Autodesk Inventor part; units mm, degrees
ref_plane "YZ Plane" through (0, 0, 0) normal (1, 0, 0) x (0, 1, 0)
ref_plane "XZ Plane" through (0, 0, 0) normal (0, 1, 0) x (-1, 0, 0)
ref_plane "XY Plane" through (0, 0, 0) normal (0, 0, 1) x (1, 0, 0)
sketch "Эскиз1" plane through (0, 0, 0) normal (0, 0, 1) x (1, 0, 0)
  line L0 (0, 0) -> (-38, 0) construction
  line L1 (-38, 0) -> (-38, 25) construction
  line L2 (-38, 25) -> (0, 25) construction
  line L3 (0, 25) -> (0, 0) construction
  line L4 (-38, 25) -> (-35, 25) construction
  line L5 (-35, 25) -> (-35, 23.5) construction
  line L6 (-35, 23.5) -> (-38, 23.5) construction
  line L7 (-38, 23.5) -> (-38, 25) construction
  line L8 (-35, 23.5) -> (-23.7, 23.5)
  line L9 (-23.7, 23.5) -> (-23.7, 3.2)
  line L10 (-23.7, 3.2) -> (-35, 3.2)
  line L11 (-35, 3.2) -> (-35, 23.5)
  line L12 (-35, 25) -> (-35, 25.3) construction
  line L13 (-35, 25.3) -> (-38, 25.3) construction
  line L14 (-35, 23.5) -> (-36, 23.5) construction
  line L15 (-36, 23.5) -> (-36, 24.5) construction
  line L16 (-36, 24.5) -> (-35, 24.5) construction
  line L17 (-35, 24.5) -> (-35, 23.5) construction
  line L18 (-36, 24.5) -> (-22.7, 24.5)
  line L19 (-22.7, 24.5) -> (-22.7, 3.2)
  line L20 (-22.7, 3.2) -> (-36, 3.2)
  line L21 (-36, 3.2) -> (-36, 24.5)
  line L22 (-38, 25.3) -> (-19.7, 25.3)
  line L23 (-19.7, 25.3) -> (-19.7, 3.2)
  line L24 (-19.7, 3.2) -> (-38, 3.2)
  line L25 (-38, 3.2) -> (-38, 25.3)
  line L26 (-23.7, 23.5) -> (-35, 23.5) construction
  line L27 (-35, 23.5) -> (-35, 17.74) construction
  line L28 (-35, 17.74) -> (-23.7, 17.74) construction
  line L29 (-23.7, 17.74) -> (-23.7, 23.5) construction
  circle A0 centre (-29.35, 17.74) radius 4.25
  line L30 (-19.7, 3.2) -> (-12.7, 3.2)
  line L31 (-12.7, 3.2) -> (-12.7, 10.2)
  line L32 (-12.7, 10.2) -> (-19.7, 10.2)
  line L33 (-19.7, 10.2) -> (-19.7, 3.2)
  line L34 (-16.2, 10.2) -> (-16.2, 3.2) construction
  line L35 (-12.7, 6.7) -> (-19.7, 6.7) construction
  circle A1 centre (-16.2, 6.7) radius 2.1
  line L36 (-29.35, 17.74) -> (-29.35, 18.74)
  point P0 (-23.7, 3.2)
  dimension "d0" = 38
  dimension "d1" = 25
  dimension "d2" = 3
  dimension "d3" = 1.5
  dimension "d4" = 11.3
  dimension "d5" = 20.3
  dimension "d6" = 0.3
  dimension "d7" = 1
  dimension "d8" = 1
  dimension "d9" = 13.3
  dimension "d10" = 21.3
  dimension "d11" = 18.3
  dimension "d12" = 5.76
  dimension "d13" = 8.5
  dimension "d19" = 7
  dimension "d20" = 7
  dimension "d21" = 4.2
  dimension "d27" = 1
extrude "Выдавливание1" add sketch "Эскиз1" along normal blind 27 contours L24 L25 L22 L23 L19 L18 L21
extrude "Выдавливание2" add sketch "Эскиз1" against normal blind 2 from surface at 27 contours L11 L20 L21 L18 L19 L9 L8 | L8 L9 L10 L11
fillet "Сопряжение1" radius 2 3 edges at (-38, 14.25, 27) (-28.85, 25.3, 27) (-19.7, 14.25, 27)
extrude "Выдавливание3" add sketch "Эскиз1" along normal blind 8 contours L23 L32 L31 L30 | A1
extrude "Выдавливание4" cut sketch "Эскиз1" along normal blind 6 contours A1
fillet "Сопряжение2" radius 2 3 edges at (-12.7, 10.2, 4) (-12.7, 3.2, 4) (-19.7, 6.7, 8)
properties part number "fast_switch"
Part model, mm, in its own coordinate system. A direction names the side the tool comes from. Round coordinates to 2 decimals unless told otherwise and drop trailing zeros. Write each loop counter-clockwise with the first axis right and the second up, starting at its lowest first coordinate (ties: lowest second). Pieces come first, ordered by that corner, then holes. Notation, with made-up numbers: M 85,-28.75 L 128,-28.75 A37 cw 128,8.25 Z; hole C -3,88 d9. An arc over 180 degrees is marked long. One line per question, with ' | ' between items.
(1) 3-axis set-ups, long thin cutter, end or side, ignore diameter. For faces 1 (the face through (-15, 7, 8)), 2 (the face through (-29, 24.5, 12)), 3 (the face through (-29, 13, 27)): which of +Z, -Z, +X, -X, +Y, -Y reach the whole face in a straight line?
Answer key:
face 1: +Z, +X, +Y, -Y | face 2: -Z, -Y | face 3: +Z, +X, -X, +Y, -Y
(2) Saw through at D-D on y = 6.7. Write the cut outline in (x, z), then the cut area to 3 significant figures.
Answer key:
outline: M -38,0 L -36,0 L -36,25 L -22.7,25 L -22.7,0 L -18.3,0 L -18.3,6 L -14.1,6 L -14.1,0 L -12.7,0 L -12.7,8 L -17.7,8 A2 cw -19.7,10 L -19.7,25 A2 ccw -21.7,27 L -36,27 A2 ccw -38,25 Z | area: 192 mm^2
(3) Pin check, flat tips, straight feed: pin 1 (6 mm diameter, centred on x = -35, y = 8, fed in from -Z); pin 2 (12 mm diameter, centred on y = 8.5, z = 22, fed in from +X); pin 3 (1.5 mm diameter, centred on x = -15.5, y = 5, fed in from +Z); pin 4 (2 mm diameter, centred on x = -15.5, y = 6, fed in from -Z). Stop position of each tip, or through.
Answer key:
pin 1: stops at z = 0 | pin 2: stops at x = -19.7 | pin 3: stops at z = 8 | pin 4: stops at z = 6
(4) Saw through at C-C on y = 17.74. Write the cut outline in (x, z), then the cut area to 3 significant figures.
Answer key:
outline: M -38,0 L -36,0 L -36,25 L -33.6,25 L -33.6,27 L -36,27 A2 ccw -38,25 Z; M -25.1,25 L -22.7,25 L -22.7,0 L -19.7,0 L -19.7,25 A2 ccw -21.7,27 L -25.1,27 Z | area: 143 mm^2
(5) Saw through at A-A on z = 3.5. Write the cut outline in (x, y), then the cut area to 3 significant figures.
Answer key:
outline: M -38,3.2 L -36,3.2 L -36,24.5 L -22.7,24.5 L -22.7,3.2 L -14.7,3.2 A2 ccw -12.7,5.2 L -12.7,8.2 A2 ccw -14.7,10.2 L -19.7,10.2 L -19.7,25.3 L -38,25.3 Z; hole C -16.2,6.7 d4.2 | area: 155 mm^2
(6) Probe line 1 along X through (y, z) = (5.25, 20.75); line 2 along Y through (x, z) = (-16.2, 2.8); line 3 along Y through (x, z) = (-27, 16.25). List the from-to ranges inside material, lowest first.
Answer key:
line 1: x = -38 to -36, -22.7 to -19.7 | line 2: y = 3.2 to 4.6, 8.8 to 10.2 | line 3: y = 24.5 to 25.3
(7) Two-plate mould, pull along Y, no slides. Class faces 4 (the face through (-22, 3.2, 14)), 5 (the face through (-32.72, 15.15, 26.01)), 6 (the face through (-36, 14, 12)), 7 (the face through (-17.866, 7.978, 2.958)): released by +Y, released by -Y, zero draft, split by the parting line, or undercut.
Answer key:
face 4: released by -Y | face 5: undercut | face 6: zero draft | face 7: undercut
(8) Saw through at B-B on x = -29.35. Write the cut outline in (y, z).
Answer key:
outline: M 3.2,25 L 13.49,25 L 13.49,27 L 3.2,27 Z; M 21.99,25 L 24.5,25 L 24.5,0 L 25.3,0 L 25.3,25 A2 ccw 23.3,27 L 21.99,27 Z
